Verification items for the finished model (mm, model axes). Round coordinates to 2 decimals unless told otherwise and drop trailing zeros. Write each loop counter-clockwise with the first axis right and the second up, starting at its lowest first coordinate (ties: lowest second). Pieces come first, ordered by that corner, then holes. Notation, with made-up numbers: M 18,-22.5 L 54,-22.5 A32 ccw 54,8.5 Z; hole C 78.5,-21.75 d1. An arc over 180 degrees is marked long. One line per question, with ' | ' between items.
Autodesk Inventor part; units mm, degrees
ref_plane "YZ Plane" through (0, 0, 0) normal (1, 0, 0) x (0, 1, 0)
ref_plane "XZ Plane" through (0, 0, 0) normal (0, 1, 0) x (-1, 0, 0)
ref_plane "XY Plane" through (0, 0, 0) normal (0, 0, 1) x (1, 0, 0)
sketch "Sketch1" plane through (0, 0, 0) normal (0, 1, 0) x (-1, 0, 0)
  line L0 (0, 0) -> (-106.68, 0)
  line L1 (-106.68, 0) -> (-106.68, -12.7)
  line L2 (-106.68, -12.7) -> (0, -12.7)
  line L3 (0, -12.7) -> (0, 0)
  dimension "d0" = 106.68
  dimension "d1" = 12.7
extrude "Extrusion1" add sketch "Sketch1" along normal blind 2.54
fillet "Fillet1" radius 3.175 4 edges at (106.68, 1.27, 0) (106.68, 1.27, -12.7) (0, 1.27, 0) (0, 1.27, -12.7)
sketch "Sketch2" plane through (0, 2.54, 0) normal (0, 1, 0) x (1, 0, 0)
  line L0 (106.68, 3.175) -> (106.68, 9.525)
  line L1 (106.68, 6.35) -> (99.06, 6.35)
  line L2 (0, 6.35) -> (7.62, 6.35)
  circle A0 centre (99.06, 6.35) radius 3.81
  circle A1 centre (7.62, 6.35) radius 3.81
  point P0 (0, 0)
  dimension "d5" = 7.62
  dimension "d6" = 7.62
  dimension "d7" = 7.62
  dimension "d8" = 7.62
extrude "Extrusion2" cut sketch "Sketch2" against normal blind 2.54 contours A0
sketch "Sketch3" plane through (0, 2.54, 0) normal (0, 1, 0) x (1, 0, 0)
  line L0 (0, 9.525) -> (0, 3.175)
  line L1 (0, 6.35) -> (7.62, 6.35)
  circle A0 centre (7.62, 6.35) radius 3.81
  point P0 (0, 0)
  dimension "d11" = 7.62
  dimension "d12" = 7.62
hole "Hole1" at (7.62, 2.54, -6.35) direction (0, -1, 0) diameter 7.62 end through all
properties part number "Side Rod V1"
1. Thickness scan on line 1 (X direction, y = 1.4, z = -6.35); line 2 (X direction, y = 1.3, z = -8); line 3 (Z direction, x = 7.62, y = 1.35). Record the ranges inside material, lowest first.
Results:
line 1: x = 0 to 3.81, 11.43 to 95.25, 102.87 to 106.68 | line 2: x = 0 to 4.19, 11.05 to 95.63, 102.49 to 106.68 | line 3: z = -12.7 to -10.16, -2.54 to 0
2. Go/stop test with a flat-tipped pin: P1, Ø1, axis at y = 0.5, z = -9.5, coming from the -X side. Record where the tip stops, or that it passes through.
Results:
P1: stops at x = 0
3. Section check A-A, the plane y = 0.6. Record the cut outline in (x, z) (3 decimals).
Results:
outline: M 0,-9.525 A3.175 ccw 3.175,-12.7 L 103.505,-12.7 A3.175 ccw 106.68,-9.525 L 106.68,-3.175 A3.175 ccw 103.505,0 L 3.175,0 A3.175 ccw 0,-3.175 Z; hole C 7.62,-6.35 d7.62; hole C 99.06,-6.35 d7.62
4. Mould release check, pull along Z, two halves, no side actions. Record for faces 1 (the face through (4.41, 1.25, -4.3)), 2 (the face through (0.91, 1.29, -0.95)), 3 (the face through (54, 0, -6)): pulls with the +Z half, pulls with the -Z half, needs draft (parallel to the pull), parting line crosses it, or undercut.
Results:
face 1: undercut | face 2: pulls with the +Z half | face 3: needs draft
5. Section check B-B, the plane z = -6.35. Record the cut outline in (x, y), then the cut area to 3 significant figures.
Results:
outline: M 0,0 L 3.81,0 L 3.81,2.54 L 0,2.54 Z; M 11.43,0 L 95.25,0 L 95.25,2.54 L 11.43,2.54 Z; M 102.87,0 L 106.68,0 L 106.68,2.54 L 102.87,2.54 Z | area: 232 mm2
6. Section check C-C, the plane x = 7.62. Record the cut outline in (y, z).
Results:
outline: M 0,-12.7 L 2.54,-12.7 L 2.54,-10.16 L 0,-10.16 Z; M 0,-2.54 L 2.54,-2.54 L 2.54,0 L 0,0 Z
